from build123d import *

# Parameters (mm, degrees)
BOSS_EXTRUDE1_DEPTH  = 6.35
SKETCH2_R            = 10.033
CUT_EXTRUDE1_DEPTH   = 9.525
SKETCH3_W            = 39.878
SKETCH3_H            = 39.878
SKETCH3_W_2          = 51.829351428
SKETCH3_H_2          = 50.992938467
CUT_EXTRUDE2_DEPTH   = 315.37310238
FILLET1_R            = 2.54
M3_CLEARANCE_HOLE1_D = 3.4
SKETCH6_R            = 19.05
CUT_EXTRUDE3_DEPTH   = 315.37310238


with BuildPart() as part:
    # Sketch1 → Boss-Extrude1 (new body)
    with BuildSketch(Plane(origin=(0, 0, 0), x_dir=(1, 0, 0), z_dir=(0, 1, 0))):
        Polygon((212.725, -212.725), (212.725, 212.725), (-212.725, 212.725), (-212.725, -9.525), (-222.25, -9.525), (-222.25, -222.25), (-9.525, -222.25), (-9.525, -212.725), align=None)
    extrude(amount=BOSS_EXTRUDE1_DEPTH)

    # Sketch2 → Cut-Extrude1 (cut)
    with BuildSketch(Plane(origin=(0, 6.35, 0), x_dir=(1, 0, 0), z_dir=(0, 1, 0))):
        with Locations(Location((-111.125, -111.125, 0), (0, 0, 270))):
            Circle(SKETCH2_R)
    extrude(amount=-CUT_EXTRUDE1_DEPTH, mode=Mode.SUBTRACT)

    # Sketch3 → Cut-Extrude2 (cut, through all)
    with BuildSketch(Plane(origin=(0, 6.35, 0), x_dir=(1, 0, 0), z_dir=(0, 1, 0))):
        with Locations((-192.786, 192.786)):
            Rectangle(SKETCH3_W, SKETCH3_H)
        with Locations((192.786, 192.786)):
            Rectangle(SKETCH3_W, SKETCH3_H)
        with Locations((192.786, -192.786)):
            Rectangle(SKETCH3_W, SKETCH3_H)
        with Locations((-198.761675714, -198.343469234)):
            Rectangle(SKETCH3_W_2, SKETCH3_H_2)
    extrude(amount=-CUT_EXTRUDE2_DEPTH, mode=Mode.SUBTRACT)

    # Fillet1
    fillet1_edges = [part.edges().sort_by_distance(p)[0] for p in [
        (-9.525, 3.175, 212.725),
        (-9.525, 3.175, 222.25),
        (-222.25, 3.175, 9.525),
        (-212.725, 3.175, 9.525),
        (-212.725, 3.175, -172.847),
        (-172.847, 3.175, -212.725),
        (-172.847, 3.175, -172.847),
        (212.725, 3.175, -172.847),
        (172.847, 3.175, -172.847),
        (172.847, 3.175, -212.725),
        (212.725, 3.175, 172.847),
        (172.847, 3.175, 212.725),
        (172.847, 3.175, 172.847),
        (-172.847, 3.175, 222.25),
        (-172.847, 3.175, 172.847),
        (-222.25, 3.175, 172.847),
    ]]
    fillet(fillet1_edges, radius=FILLET1_R)

    # M3 Clearance Hole1 (through all)
    with Locations(Plane(origin=(0, 6.35, 0), x_dir=(1, 0, 0), z_dir=(0, 1, 0))):
        with Locations((-164.211, -193.421), (-193.421, -164.211), (-193.421, 164.211), (-164.211, 193.421), (164.211, 193.421), (193.421, 164.211), (193.421, -164.211), (164.211, -193.421)):
            Hole(M3_CLEARANCE_HOLE1_D / 2)

    # Sketch6 → Cut-Extrude3 (cut, through all)
    with BuildSketch(Plane(origin=(0, 6.35, 0), x_dir=(1, 0, 0), z_dir=(0, 1, 0))):
        with Locations(Location((-195.453, -132.969, 0), (0, 0, 270))):
            Circle(SKETCH6_R)
        with Locations(Location((-132.969, -195.453, 0), (0, 0, 270))):
            Circle(SKETCH6_R)
        with BuildLine():
            ThreePointArc((-184.342788517, -156.794925413), (-180.374249065, -154.503688092), (-176.863869829, -151.558130171))
            ThreePointArc((-176.863869829, -151.558130171), (-176.863869829, -148.325237967), (-180.096762033, -148.325237967))
            ThreePointArc((-180.096762033, -148.325237967), (-182.996640532, -150.758524946), (-186.27499921, -152.651286211))
            ThreePointArc((-186.27499921, -152.651286211), (-187.380713465, -155.689211159), (-184.342788517, -156.794925413))
        make_face()
        with BuildLine():
            ThreePointArc((-110.20205816, -182.3085), (-112.112534037, -179.449270793), (-114.379869829, -176.863869829))
            ThreePointArc((-114.379869829, -176.863869829), (-117.612762033, -176.863869829), (-117.612762033, -180.096762033))
            ThreePointArc((-117.612762033, -180.096762033), (-115.739745509, -182.232528046), (-114.161526306, -184.5945))
            ThreePointArc((-114.161526306, -184.5945), (-111.038792233, -185.431234073), (-110.20205816, -182.3085))
        make_face()
        with BuildLine():
            ThreePointArc((-219.278925413, -144.079211483), (-216.987688092, -148.047750935), (-214.042130171, -151.558130171))
            ThreePointArc((-214.042130171, -151.558130171), (-210.809237967, -151.558130171), (-210.809237967, -148.325237967))
            ThreePointArc((-210.809237967, -148.325237967), (-213.242524946, -145.425359468), (-215.135286211, -142.14700079))
            ThreePointArc((-215.135286211, -142.14700079), (-218.173211159, -141.041286535), (-219.278925413, -144.079211483))
        make_face()
        with BuildLine():
            ThreePointArc((-206.563211483, -109.143074587), (-210.531750935, -111.434311908), (-214.042130171, -114.379869829))
            ThreePointArc((-214.042130171, -114.379869829), (-214.042130171, -117.612762033), (-210.809237967, -117.612762033))
            ThreePointArc((-210.809237967, -117.612762033), (-207.909359468, -115.179475054), (-204.63100079, -113.286713789))
            ThreePointArc((-204.63100079, -113.286713789), (-203.525286535, -110.248788841), (-206.563211483, -109.143074587))
        make_face()
        with BuildLine():
            ThreePointArc((-171.627074587, -121.858788517), (-173.918311908, -117.890249065), (-176.863869829, -114.379869829))
            ThreePointArc((-176.863869829, -114.379869829), (-180.096762033, -114.379869829), (-180.096762033, -117.612762033))
            ThreePointArc((-180.096762033, -117.612762033), (-177.663475054, -120.512640532), (-175.770713789, -123.79099921))
            ThreePointArc((-175.770713789, -123.79099921), (-172.732788841, -124.896713465), (-171.627074587, -121.858788517))
        make_face()
        with BuildLine():
            ThreePointArc((-119.8245, -218.21994184), (-116.965270793, -216.309465963), (-114.379869829, -214.042130171))
            ThreePointArc((-114.379869829, -214.042130171), (-114.379869829, -210.809237967), (-117.612762033, -210.809237967))
            ThreePointArc((-117.612762033, -210.809237967), (-119.748528046, -212.682254491), (-122.1105, -214.260473694))
            ThreePointArc((-122.1105, -214.260473694), (-122.947234073, -217.383207767), (-119.8245, -218.21994184))
        make_face()
        with BuildLine():
            ThreePointArc((-155.73594184, -208.5975), (-153.825465963, -211.456729207), (-151.558130171, -214.042130171))
            ThreePointArc((-151.558130171, -214.042130171), (-148.325237967, -214.042130171), (-148.325237967, -210.809237967))
            ThreePointArc((-148.325237967, -210.809237967), (-150.198254491, -208.673471954), (-151.776473694, -206.3115))
            ThreePointArc((-151.776473694, -206.3115), (-154.899207767, -205.474765927), (-155.73594184, -208.5975))
        make_face()
        with BuildLine():
            ThreePointArc((-146.1135, -172.68605816), (-148.972729207, -174.596534037), (-151.558130171, -176.863869829))
            ThreePointArc((-151.558130171, -176.863869829), (-151.558130171, -180.096762033), (-148.325237967, -180.096762033))
            ThreePointArc((-148.325237967, -180.096762033), (-146.189471954, -178.223745509), (-143.8275, -176.645526306))
            ThreePointArc((-143.8275, -176.645526306), (-142.990765927, -173.522792233), (-146.1135, -172.68605816))
        make_face()
    extrude(amount=-CUT_EXTRUDE3_DEPTH, mode=Mode.SUBTRACT)


solid = part.part
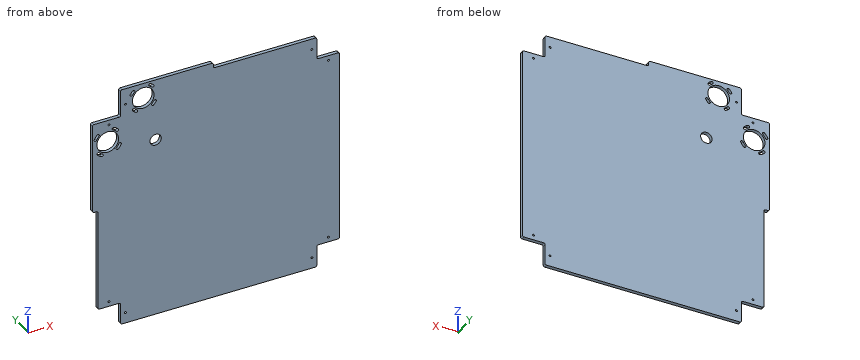
Here's how the part is built. I have some questions about the finished solid (model axes, mm). Give positions to 0.01 mm unless a question says otherwise; leave off trailing zeros. Loops run counter-clockwise (first coordinate to the right, second up) from the corner with the lowest first, then second, coordinate; pieces in that order, holes last. Notation, with made-up numbers: (55, -4) -> (92, -4) arc R13 cw to (92, 7) -> close; hole circle Ø4 at (12.25, 56.5). An arc over 180 degrees is marked (long way). One line per item, written item: value.
Q1. I'm going to push flat-ended pins straight in: pin 1 Ø3 at (y, z) = (3.5, 186) entering from +X; pin 2 Ø2 at (x, y) = (-8, 5.5) entering from +Z; pin 3 Ø1.3 at (y, z) = (3.5, 217) entering from +X (3 decimals). Where does each tip first touch, or does it pass through?
Answers follow:
pin 1: x = 172.85
pin 2: z = 213.72
pin 3: x = -9.525
Q2. Suppose I cut it at B-B on x = 66.5. Please give me the cut outline in (y, z) (3 decimals).
Answers follow:
outline: (0, -212.725) -> (6.35, -212.725) -> (6.35, 212.725) -> (0, 212.725) -> close
Q3. If I drill on line 1 along X through (y, z) = (2.5, 193.5); line 2 along Z through (x, y) = (11, 1) (3 decimals), over which ranges is the centre line in solid material (lowest first)?
Answers follow:
line 1: -172.85 to -165.91, -162.51 to -151.92, -114.02 to 162.51, 165.91 to 172.85
line 2: -212.725 to 212.725
Q4. Suppose I cut it at A-A on z = -130. Please give me the cut outline in (x, y) (3 decimals), then the cut area to 3 significant figures.
Answers follow:
outline: (-212.725, 0) -> (212.725, 0) -> (212.725, 6.35) -> (-212.725, 6.35) -> close
area: 2,700 mm^2
Q5. Suppose I cut it at C-C on y = 4. State how many separate pieces and enclosed holes the cut face has, then the cut area to 3 significant figures.
Answers follow:
separate pieces: 1
enclosed holes: 19
area: 175,000 mm^2
